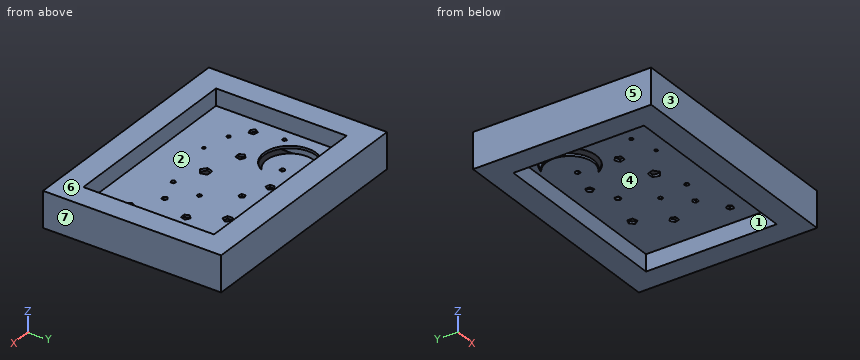
from build123d import *

# Parameters (mm, degrees)
F0_W     = 100
F0_H     = 75
F0_W_2   = 80
F0_H_2   = 55
F1_DEPTH = 7.5
F2_W     = 85
F2_H     = 60
F3_DEPTH = 0.5
F5_DEPTH = 4
F7_DEPTH = 4
F9_DEPTH = 2


with BuildPart() as f1:
    # F0 (on Top) → F1 (new body, symmetric)
    with BuildSketch(Plane.XY):
        Rectangle(F0_W, F0_H)
        Rectangle(F0_W_2, F0_H_2, mode=Mode.SUBTRACT)
    extrude(amount=F1_DEPTH, both=True)

    # F2 (on Top) → F3 (join, symmetric)
    with BuildSketch(Plane.XY):
        Rectangle(F2_W, F2_H)
    extrude(amount=F3_DEPTH, both=True)

    # F4 (on face) → F5 (cut, symmetric)
    with BuildSketch(Plane.XY.offset(0.5)):
        with BuildLine():
            ThreePointArc((-14.030779073, 9.8216604466), (-28.5453805779, 11.5757365705), (-25.4971957792, 25.8746529394))
            ThreePointArc((-25.4971957792, 25.8746529394), (-32.7417275782, 8.5783475559), (-14.030779073, 9.8216604466))
        make_face()
    extrude(amount=F5_DEPTH, both=True, mode=Mode.SUBTRACT)

    # F6 (on face) → F7 (cut, symmetric)
    with BuildSketch(Plane.XY.offset(0.5)):
        Polygon((-33.6119382633, -8.6941833252), (-31.7468941212, -8.0039128661), (-31.8270500041, -6.016845179), (-33.7416332062, -5.4790402695), (-34.8447548165, -7.1337262432), align=None)
        Polygon((-18.1541709736, -2.747406776), (-15.9509722143, -2.5300781708), (-15.4768381419, -0.3675534018), (-17.3870059292, 0.7516318018), (-19.0416886183, -0.7191984717), align=None)
        Polygon((-35.4328444953, 4.0322221243), (-34.4056151807, 4.1949180886), (-34.2429169225, 5.2221470399), (-35.1695931836, 5.6943134817), (-35.9050088677, 4.9588994397), align=None)
        Polygon((-2.2557034881, -7.8243230846), (0, -6.2835649587), (-0.7682973436, -3.6621430124), (-3.4988347035, -3.5827732766), (-4.4181022559, -6.1551420285), align=None)
        Polygon((25.5881788104, 4.9083078249), (27.6833120733, 4.9768951721), (28.2655134136, 6.9906799703), (26.5302003672, 8.1666800743), (24.8755165832, 6.8797033113), align=None)
        Polygon((19.9947226477, -7.7864271936), (21.4274991304, -7.6911230572), (21.7796117926, -6.2990210491), (20.5644529031, -5.5339588288), (19.4613307453, -6.4532263812), align=None)
        Polygon((11.3635717008, 2.5557714691), (11.4182028919, 1.3798037544), (12.5534966165, 1.068367096), (13.2005155343, 2.0518563705), (12.4651014924, 2.9711228281), align=None)
        Polygon((3.0226850162, 13.37136293), (4.5368093997, 12.9530541599), (5.4025348475, 14.2638075025), (4.4234582156, 15.4922063892), (2.9526301317, 14.9406453103), align=None)
        Polygon((19.9522579427, 20.7217878026), (17.8304072469, 19.9908427894), (17.8698893403, 17.7469684276), (20.0161413117, 17.0911228187), (21.3031158851, 18.9296623029), align=None)
        Polygon((-7.5485593761, 17.8178252237), (-5.6288838387, 17.3321217299), (-4.5737400011, 19.0077510251), (-5.8413007839, 20.529050376), (-7.6798402681, 19.7936357866), align=None)
        Polygon((-18.8396373222, 14.8832345039), (-17.5149254501, 14.8297967389), (-17.0547446343, 16.0731594196), (-18.0950491213, 16.8950375816), (-19.1981734687, 16.1596235397), align=None)
    extrude(amount=F7_DEPTH, both=True, mode=Mode.SUBTRACT)

    # F8 (on face) → F9 (cut)
    with BuildSketch(Plane.XY.offset(0.5)):
        Polygon((-26.2314461983, -12.9390526563), (-25.1804060423, -12.9390526563), (-24.8556167723, -11.9394540671), (-25.7059261203, -11.3216681638), (-26.5562354682, -11.9394540671), align=None)
        Polygon((-14.0670929104, -15.3417089426), (-14.0670929104, -14.4817656435), (-14.8849475887, -14.2160285498), (-15.3904095777, -14.911737293), (-14.8849475887, -15.6074460362), align=None)
        Polygon((32.2768948972, -14.9704083861), (32.2768948972, -13.2021199851), (30.5951526907, -12.6556888182), (29.5557788468, -14.0862641856), (30.5951526907, -15.516839553), align=None)
        Polygon((10.7780173421, -11.227759206), (10.7780173421, -10.0489047829), (9.6568601613, -9.6846187323), (8.9639469168, -10.6383319944), (9.6568601613, -11.5920452566), align=None)
    extrude(amount=-F9_DEPTH, mode=Mode.SUBTRACT)


solid = f1.part
Can you work these out from the model? Positions are in its coordinate system, mm. Face numbers are marked on the shaded views. A direction names the side the tool comes from. Coordinates: 2 decimals unless noted, no trailing zeros. Write each loop counter-clockwise with the first axis right and the second up, starting at its lowest first coordinate (ties: lowest second). Pieces come first, ordered by that corner, then holes. Notation, with made-up numbers: (52, 71) -> (78, 71) arc R17 cw to (78, 96) -> close; hole circle Ø8 at (89.25, 6.25). An arc over 180 degrees is marked (long way). Write each question's results on one line, items separated by ' | '. Start each with the question number.
Item 1: If we section it at B-B, the plane y = -18: Write out the boundary of the cut face in (x, z).
Item 2: If we section it at D-D, the plane x = 7: Write out the boundary of the cut face in (y, z), and give its area (3 significant figures).
Item 3: I'm going to push flat-ended pins straight in: P1, Ø6, axis at x = 6.5, y = 19, coming from the -Z side; P2, Ø17.5, axis at x = -23.77, y = 14.99, coming from the +Z side. Where does each tip first touch, or does it pass through?
Item 4: Please list where these lines run through material, in increasing order: probe 1 along X at (y, z) = (-20, -1.5); probe 2 along Y at (x, z) = (-16.5, 6); probe 3 along Z at (x, y) = (9, 12).
Item 5: Thinking about a two-plate mould opening in X: for the marked faces 4, 5, 6 and 7, which applies, released by +X, released by -X, zero draft, split by the parting line, or undercut?
Item 6: If we section it at C-C, the plane y = 24: Write out the boundary of the cut face in (x, z), and give its area (3 significant figures).
Item 7: If we section it at A-A, the plane z = 2: Write out the boundary of the cut face in (x, y).
Item 8: On a 3-axis mill with a long thin cutter (end or side, diameter ignored), from which of +Z, -Z, +X, -X, +Y, -Y can I reach the whole of each face in a straight line? I mean the marked faces 1, 2 and 3. Say none if no direction works.
Answer block:
1) outline: (-50, -7.5) -> (-40, -7.5) -> (-40, -0.5) -> (40, -0.5) -> (40, -7.5) -> (50, -7.5) -> (50, 7.5) -> (40, 7.5) -> (40, 0.5) -> (-40, 0.5) -> (-40, 7.5) -> (-50, 7.5) -> close
2) outline: (-37.5, -7.5) -> (-27.5, -7.5) -> (-27.5, -0.5) -> (27.5, -0.5) -> (27.5, -7.5) -> (37.5, -7.5) -> (37.5, 7.5) -> (27.5, 7.5) -> (27.5, 0.5) -> (-27.5, 0.5) -> (-27.5, 7.5) -> (-37.5, 7.5) -> close | area: 355 mm²
3) P1: z = -0.5 | P2: z = 0.5
4) probe 1: -50 to -40, 40 to 50 | probe 2: -37.5 to -27.5, 27.5 to 37.5 | probe 3: -0.5 to 0.5
5) face 4: undercut | face 5: released by -X | face 6: zero draft | face 7: released by +X
6) outline: (-50, -7.5) -> (-40, -7.5) -> (-40, -0.5) -> (-30.12, -0.5) -> (-30.12, 0.5) -> (-40, 0.5) -> (-40, 7.5) -> (-50, 7.5) -> close; (-27.81, -0.5) -> (40, -0.5) -> (40, -7.5) -> (50, -7.5) -> (50, 7.5) -> (40, 7.5) -> (40, 0.5) -> (-27.81, 0.5) -> close | area: 378 mm²
7) outline: (-50, -37.5) -> (50, -37.5) -> (50, 37.5) -> (-50, 37.5) -> close; hole (-40, -27.5) -> (40, -27.5) -> (40, 27.5) -> (-40, 27.5) -> close
8) face 1: -Z | face 2: +Z | face 3: +Z, -Z, +X, -X, -Y
